```python
from build123d import *

# Parameters (mm, degrees)
F0_W        = 18.5
F0_H        = 13
F0_W_2      = 4.3
F0_W_3      = 3
F0_H_2      = 2.95
F1_DEPTH    = 10
F3_DEPTH    = 7
F4_T1_DEPTH = 35
F4_T3_DEPTH = 34.4948974279
F0_H_3      = 5.9
F5_DEPTH    = 14
F6_R        = 5.5
F7_DEPTH    = 4
F8_SIZE     = 2


# Not quite as in the source:
# - a fillet or chamfer that OpenCascade refuses, or shapes differently, is made with other operations: its cross-section is extruded or revolved along the edge and cut away or added


with BuildPart() as f1:
    # F0 (on Top) → F1 (new body)
    with BuildSketch(Plane.XY):
        with Locations((5.190736489, 6.5)):
            Rectangle(F0_W, F0_H)
        with Locations((16.590736489, 6.5)):
            Rectangle(F0_W_2, F0_H)
        Polygon((14.440736489, 20.05), (14.440736489, 13), (18.740736489, 13), (18.740736489, 20.05), (15.740736489, 20.05), (15.740736489, 25.95), (18.740736489, 25.95), (18.740736489, 33), (14.440736489, 33), (14.440736489, 25.95), (14.440736489, 23), align=None)
        with BuildLine():
            Line((-4.059263511, 20.05), (-4.059263511, 13))
            Line((-4.059263511, 13), (14.440736489, 13))
            Line((14.440736489, 13), (14.440736489, 20.05))
            Line((14.440736489, 20.05), (11.440736489, 20.05))
            Line((11.440736489, 20.05), (11.440736489, 23))
            Line((11.440736489, 23), (9.590736489, 23))
            ThreePointArc((9.590736489, 23), (8.4904647177, 21.0659304563), (6.265736489, 21.0234183548))
            ThreePointArc((6.265736489, 21.0234183548), (4.0410082602, 21.0659304563), (2.940736489, 23))
            Line((2.940736489, 23), (-1.059263511, 23))
            Line((-1.059263511, 23), (-1.059263511, 20.05))
            Line((-1.059263511, 20.05), (-4.059263511, 20.05))
        make_face()
        with Locations((12.940736489, 21.525)):
            Rectangle(F0_W_3, F0_H_2)
        with Locations((12.940736489, 24.475)):
            Rectangle(F0_W_3, F0_H_2)
        with BuildLine():
            Line((-4.059263511, 33), (-4.059263511, 25.95))
            Line((-4.059263511, 25.95), (-1.059263511, 25.95))
            Line((-1.059263511, 25.95), (-1.059263511, 23))
            Line((-1.059263511, 23), (2.940736489, 23))
            ThreePointArc((2.940736489, 23), (4.0410082602, 24.9340695437), (6.265736489, 24.9765816452))
            ThreePointArc((6.265736489, 24.9765816452), (8.4904647177, 24.9340695437), (9.590736489, 23))
            Line((9.590736489, 23), (11.440736489, 23))
            Line((11.440736489, 23), (11.440736489, 25.95))
            Line((11.440736489, 25.95), (14.440736489, 25.95))
            Line((14.440736489, 25.95), (14.440736489, 33))
            Line((14.440736489, 33), (-4.059263511, 33))
        make_face()
        with BuildLine():
            Line((5.090736489, 23), (2.940736489, 23))
            ThreePointArc((2.940736489, 23), (4.0410082602, 21.0659304563), (6.265736489, 21.0234183548))
            ThreePointArc((6.265736489, 21.0234183548), (5.4066669452, 21.8502717712), (5.090736489, 23))
        make_face()
        with BuildLine():
            ThreePointArc((6.265736489, 24.9765816452), (4.0410082602, 24.9340695437), (2.940736489, 23))
            Line((2.940736489, 23), (5.090736489, 23))
            ThreePointArc((5.090736489, 23), (5.4066669452, 24.1497282288), (6.265736489, 24.9765816452))
        make_face()
    extrude(amount=F1_DEPTH)

    # F2 (on face) → F3 (cut)
    with BuildSketch(Plane.XZ):
        Polygon((2.840736489, 10), (0.940736489, 10), (0.940736489, 9), (1.940736489, 9), (1.940736489, 8), (0.940736489, 8), (0.940736489, 7), (1.940736489, 7), (1.940736489, 6), (0.940736489, 6), (0.940736489, 5), (1.940736489, 5), (1.940736489, 4), (0.940736489, 4), (0.940736489, 3), (1.940736489, 3), (1.940736489, 2), (0.940736489, 2), (0.940736489, 1), (1.940736489, 1), (1.940736489, 0), (2.840736489, 0), align=None)
        Polygon((14.740736489, 10), (12.840736489, 10), (12.840736489, 9), (13.840736489, 9), (13.840736489, 8), (12.840736489, 8), (12.840736489, 7), (13.840736489, 7), (13.840736489, 6), (12.840736489, 6), (12.840736489, 5), (13.840736489, 5), (13.840736489, 4), (12.840736489, 4), (12.840736489, 3), (13.840736489, 3), (13.840736489, 2), (12.840736489, 2), (12.840736489, 1), (13.840736489, 1), (13.840736489, 0), (14.740736489, 0), align=None)
    extrude(amount=-F3_DEPTH, mode=Mode.SUBTRACT)

    # F4: fillet of radius 5 on 4 edges, made by hand

    # F4_s2 → F4_t1 (cut)
    with BuildSketch(Plane.XY.offset(-12.5)):
        with BuildLine():
            ThreePointArc((-4.059263511, 28), (-2.594797417, 31.5355339059), (0.940736489, 33))
            Line((0.940736489, 33), (-4.059263511, 33))
            Line((-4.059263511, 33), (-4.059263511, 28))
        make_face()
        with BuildLine():
            ThreePointArc((0.940736489, 0), (-2.594797417, 1.4644660941), (-4.059263511, 5))
            Line((-4.059263511, 5), (-4.059263511, 0))
            Line((-4.059263511, 0), (0.940736489, 0))
        make_face()
        with BuildLine():
            ThreePointArc((13.740736489, 33), (17.2762703949, 31.5355339059), (18.740736489, 28))
            Line((18.740736489, 28), (18.740736489, 33))
            Line((18.740736489, 33), (13.740736489, 33))
        make_face()
    extrude(amount=F4_T1_DEPTH, mode=Mode.SUBTRACT)

    # F4_s4 → F4_t3 (cut)
    with BuildSketch(Plane.XY.offset(-12.2474487139)):
        with BuildLine():
            ThreePointArc((18.740736489, 4.8989794856), (17.6137198352, 1.7367018254), (14.740736489, 0))
            Line((14.740736489, 0), (18.740736489, 0))
            Line((18.740736489, 0), (18.740736489, 4.8989794856))
        make_face()
    extrude(amount=F4_T3_DEPTH, mode=Mode.SUBTRACT)

    # F0 (on Top) → F5 (join)
    with BuildSketch(Plane.XY):
        with Locations((-2.559263511, 24.475)):
            Rectangle(F0_W_3, F0_H_2)
        with Locations((-2.559263511, 21.525)):
            Rectangle(F0_W_3, F0_H_2)
        with Locations((17.240736489, 23)):
            Rectangle(F0_W_3, F0_H_3)
    extrude(amount=F5_DEPTH)

    # F6 (on face) → F7 (cut)
    with BuildSketch(Plane(origin=(0, 0, 0), x_dir=(1, 0, 0), z_dir=(0, 0, -1))):
        with Locations((7.340736489, -23)):
            Circle(F6_R)
    extrude(amount=-F7_DEPTH, mode=Mode.SUBTRACT)

    # F8
    f8_edges = [f1.edges().sort_by_distance(p)[0] for p in [
        (1.840736, 23, 4),
    ]]
    chamfer(f8_edges, length=F8_SIZE)


solid = f1.part
```
Verification items for the finished model (mm, model axes). A direction names the side the tool comes from. Coordinates: 2 decimals unless noted, no trailing zeros. Order: outer loops, then holes, each group sorted by start corner. A loop starts at its lowest first (then second) coordinate and runs counter-clockwise, first axis right, second up. Notation, with made-up numbers: (34, -19.5) -> (57, -19.5) arc R24 cw to (57, 16.5) -> close; hole circle Ø4 at (59, 89). An arc over 180 degrees is marked (long way). Put each result on its own line as item: value. Start each with the question number.
1) Tool access check on faces 1 (the flat face through (15.741, 23, 12)), 2 (the flat face through (12.841, 3.5, 9.5)), 3 (the flat face through (13, 3, 5)), 4 (the flat face through (1.4, 0, 6.5)), 5 (the flat face through (1.941, 3.5, 2.5)). Record the directions out of +Z, -Z, +X, -X, +Y, -Y that give a thin tool (end or side, any length) a straight path to the whole face; none if there is none.
2) Release check for a two-part mould opening along X. For faces 6 (the cylindrical face through (17.24, 31.57, 4.93)), 7 (the flat face through (1.4, 3.5, 8)), 8 (the flat face through (8, 0, 5)) record: pulls with the +X half, pulls with the -X half, needs draft (parallel to the pull), parting line crosses it, or undercut.
3) Material ranges on L1, parallel to Z at x = 13.5, y = 2.5; L2, parallel to X at y = 23, z = 0.65; L3, parallel to X at y = 25, z = 11.75, recorded low to high.
4) Cross-section at B-B (y = 4). State how many separate pieces and enclosed holes the cut face has, plus the area to 3 significant figures.
5) Cross-section at C-C (y = 16). Enter the section's corners in (x, z).
6) Cross-section at D-D (y = 31.5). Enter the section's corners in (x, z), plus the area to 3 significant figures.
7) Cross-section at A-A (z = 7.5). Enter the section's corners in (x, y).
8) Go/stop test with flat-tipped pins: pin 1 (4 mm diameter, centred on x = 13.5, y = 6.5, fed in from +Z); pin 2 (0.8 mm diameter, centred on x = 1.5, y = 3.5, fed in from -Z); pin 3 (0.8 mm diameter, centred on y = 2.5, z = 7.5, fed in from +X); pin 4 (1.1 mm diameter, centred on y = 4, z = 8.5, fed in from +X). Record where each tip stops, or that it passes through.
Geometry check:
1. face 1: +Z, +Y, -Y
1. face 2: +Z, -Y
1. face 3: -Y
1. face 4: +Z, -Z, +X, -X, -Y
1. face 5: +Z, -Z, -Y
2. face 6: pulls with the +X half
2. face 7: undercut
2. face 8: needs draft
3. L1: z = 0 to 1, 2 to 3, 4 to 5, 6 to 7, 8 to 9
3. L2: x = -4.06 to 1.84, 12.84 to 18.74
3. L3: x = -4.06 to -1.06, 15.74 to 18.74
4. separate pieces: 3
4. enclosed holes: 0
4. area: 198 mm^2
5. outline: (-4.06, 0) -> (18.74, 0) -> (18.74, 10) -> (-4.06, 10) -> close
6. outline: (-2.63, 0) -> (17.31, 0) -> (17.31, 10) -> (-2.63, 10) -> close
6. area: 199 mm^2
7. outline: (-4.06, 5) arc R5 ccw to (0.94, 0) -> (0.94, 7) -> (2.84, 7) -> (2.84, 0) -> (12.84, 0) -> (12.84, 7) -> (14.74, 7) -> (14.74, 0) arc R5 ccw to (18.74, 4.9) -> (18.74, 28) arc R5 ccw to (13.74, 33) -> (0.94, 33) arc R5 ccw to (-4.06, 28) -> close; hole circle Ø4.5 at (7.34, 23)
8. pin 1: stops at z = 10
8. pin 2: stops at z = 0
8. pin 3: stops at x = 18.32
8. pin 4: stops at x = 18.73
